from build123d import *

# Parameters (mm, degrees)
BOSS_EXTRUDE1_DEPTH = 10
CUT_EXTRUDE1_DEPTH  = 1
CHAMFER1_SIZE       = 1
CUT_EXTRUDE2_DEPTH  = 6


with BuildPart() as part:
    # Sketch2 → Boss-Extrude1 (new body)
    with BuildSketch(Plane(origin=(0, 0, 0), x_dir=(1, 0, 0), z_dir=(0, 1, 0))):
        with BuildLine():
            Line((-13.742133053, -2.045066795), (-2.112067201, -2.853361551))
            ThreePointArc((-2.112067201, -2.853361551), (0, -3.55), (2.112067201, -2.853361551))
            Line((2.112067201, -2.853361551), (13.742133053, -2.045066795))
            ThreePointArc((13.742133053, -2.045066795), (15.65, 0), (13.742133053, 2.045066795))
            Line((13.742133053, 2.045066795), (2.112067201, 2.853361551))
            ThreePointArc((2.112067201, 2.853361551), (0, 3.55), (-2.112067201, 2.853361551))
            Line((-2.112067201, 2.853361551), (-13.742133053, 2.045066795))
            ThreePointArc((-13.742133053, 2.045066795), (-15.65, 0), (-13.742133053, -2.045066795))
        make_face()
    extrude(amount=BOSS_EXTRUDE1_DEPTH)

    # Sketch3 → Cut-Extrude1 (cut)
    with BuildSketch(Plane.XZ):
        with BuildLine():
            ThreePointArc((-2.112067201, 2.853361551), (0, -3.55), (2.112067201, 2.853361551))
            ThreePointArc((2.112067201, 2.853361551), (0, 3.55), (-2.112067201, 2.853361551))
        make_face()
    extrude(amount=-CUT_EXTRUDE1_DEPTH, mode=Mode.SUBTRACT)

    # Chamfer1
    chamfer1_edges = [part.edges().sort_by_distance(p)[0] for p in [
        (3.55, 0, 0),
        (-3.55, 0, 0),
    ]]
    chamfer(chamfer1_edges, length=CHAMFER1_SIZE - 0.0001)  # a hair under: the kernel refuses the full size

    # Shaft Key → Cut-Extrude2 (cut)
    with BuildSketch(Plane(origin=(0, 10, 0), x_dir=(1, 0, 0), z_dir=(0, 1, 0))):
        with BuildLine():
            Line((1.6, -1.855397532), (1.6, -5.45))
            Line((1.6, -5.45), (-1.6, -5.45))
            Line((-1.6, -5.45), (-1.6, -1.855397532))
            ThreePointArc((-1.6, -1.855397532), (-2.45, 0), (-1.6, 1.855397532))
            Line((-1.6, 1.855397532), (-1.6, 5.45))
            Line((-1.6, 5.45), (1.6, 5.45))
            Line((1.6, 5.45), (1.6, 1.855397532))
            ThreePointArc((1.6, 1.855397532), (2.45, 0), (1.6, -1.855397532))
        make_face()
    extrude(amount=-CUT_EXTRUDE2_DEPTH, mode=Mode.SUBTRACT)


solid = part.part
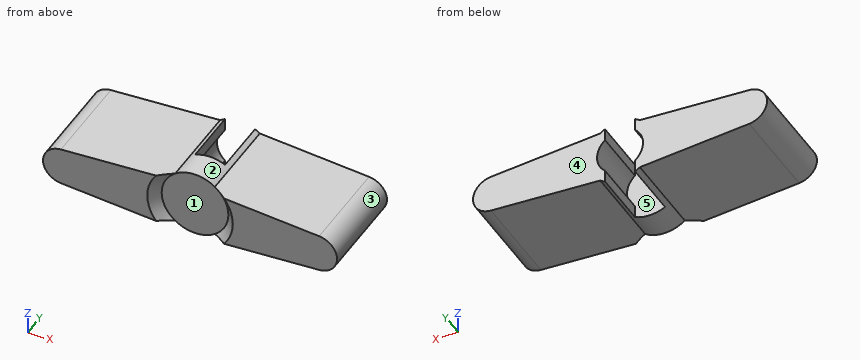
Here's how the part is built. I have some questions about the finished solid (model axes, mm). Face numbers are marked on the shaded views. A direction names the side the tool comes from. Coordinates: 2 decimals unless noted, no trailing zeros. Write each loop counter-clockwise with the first axis right and the second up, starting at its lowest first coordinate (ties: lowest second). Pieces come first, ordered by that corner, then holes.
Item 1: If I drill on line 1 (Z direction, x = 8, y = 1); line 2 (Y direction, x = -1, z = 1.5); line 3 (X direction, y = 9, z = -1.5), over which ranges is the centre line in solid material (lowest first)?
Item 2: I want a section at C-C on x = -7.5. Write out the boundary of the cut face in (y, z).
Item 3: Will these pins go through, and if not, where does the flat tip stop? pin 1 (1.1 mm diameter, centred on y = 7.5, z = -2, fed in from -X); pin 2 (3 mm diameter, centred on y = 2, z = 2.5, fed in from +X); pin 3 (1 mm diameter, centred on x = 3, y = 7.5, fed in from +Z).
Item 4: On a 3-axis mill with a long thin cutter (end or side, diameter ignored), from which of +Z, -Z, +X, -X, +Y, -Y can I reach the whole of each face in a straight line? I mean the marked faces 4 and 5. Say none if no direction works.
Item 5: If we mould it in two halves opening along Z, with no side actions, what happens to the marked faces 1, 2 and 3? For each: +Z half, -Z half, draft (parallel to the pull), parting line (faces both ways), or undercut.
Item 6: I want a section at D-D on x = 8.5. Write out the boundary of the cut face in (y, z).
Findings below:
1. line 1: z = -2.44 to 2.44
1. line 2: y = 1 to 4
1. line 3: x = -15 to -1.94, 1.94 to 15
2. outline: (0, -2.48) - (10, -2.48) - (10, 2.48) - (0, 2.48) - close
3. pin 1: stops at x = -15.05
3. pin 2: stops at x = 15.39
3. pin 3: stops at z = 2.83
4. face 4: +Z, -Z, +X, -X, +Y
4. face 5: +Y
5. face 1: undercut
5. face 2: +Z half
5. face 3: parting line
6. outline: (0, -2.41) - (10, -2.41) - (10, 2.41) - (0, 2.41) - close
